Build history of the part. All positions in model axes, mm. A direction names the side the tool comes from. Coordinates: 2 decimals unless noted, no trailing zeros. Order: outer loops, then holes, each group sorted by start corner. A loop starts at its lowest first (then second) coordinate and runs counter-clockwise, first axis right, second up. Notation, with made-up numbers: (64.25, 54.25) - (76.25, 54.25) arc R6 ccw to (76.25, 64.25) - close; hole circle Ø8 at (-5.75, 49.5). An arc over 180 degrees is marked (long way). Write each question's results on one line, items separated by ' | '. Start each with the question number.
from build123d import *

# Parameters (mm, degrees)
SKETCH1_W           = 200
SKETCH1_H           = 78
BOSS_EXTRUDE1_DEPTH = 4
SKETCH2_W           = 35
SKETCH2_H           = 4
CUT_EXTRUDE1_DEPTH  = 4
CUT_EXTRUDE2_DEPTH  = 4


with BuildPart() as part:
    # Sketch1 → Boss-Extrude1 (new body)
    with BuildSketch(Plane.XY):
        with Locations((-100, 39)):
            Rectangle(SKETCH1_W, SKETCH1_H)
    extrude(amount=BOSS_EXTRUDE1_DEPTH)

    # Sketch2 → Cut-Extrude1 (cut)
    with BuildSketch(Plane.XY.offset(4)):
        with Locations((-182.5, 76)):
            Rectangle(SKETCH2_W, SKETCH2_H)
        with Locations((-127.5, 76)):
            Rectangle(SKETCH2_W, SKETCH2_H)
        with Locations((-72.5, 76)):
            Rectangle(SKETCH2_W, SKETCH2_H)
        with Locations((-17.5, 76)):
            Rectangle(SKETCH2_W, SKETCH2_H)
        with Locations((-182.5, 2)):
            Rectangle(SKETCH2_W, SKETCH2_H)
        with Locations((-127.5, 2)):
            Rectangle(SKETCH2_W, SKETCH2_H)
        with Locations((-72.5, 2)):
            Rectangle(SKETCH2_W, SKETCH2_H)
        with Locations((-17.5, 2)):
            Rectangle(SKETCH2_W, SKETCH2_H)
    extrude(amount=-CUT_EXTRUDE1_DEPTH, mode=Mode.SUBTRACT)

    # Sketch4 → Cut-Extrude2 (cut)
    with BuildSketch(Plane.XY.offset(4)):
        Polygon((-125.75, 74), (-129.25, 74), (-129.25, 70.25), (-130.5, 70.25), (-130.5, 67.75), (-129.25, 67.75), (-129.25, 64), (-125.75, 64), (-125.75, 67.75), (-124.5, 67.75), (-124.5, 70.25), (-125.75, 70.25), align=None)
        Polygon((-70.75, 67.75), (-69.5, 67.75), (-69.5, 70.25), (-70.75, 70.25), (-70.75, 74), (-74.25, 74), (-74.25, 70.25), (-75.5, 70.25), (-75.5, 67.75), (-74.25, 67.75), (-74.25, 64), (-70.75, 64), align=None)
    extrude(amount=-CUT_EXTRUDE2_DEPTH, mode=Mode.SUBTRACT)


solid = part.part
Item 1: Which spindle directions (+Z, -Z, +X, -X, +Y, -Y) get a long thin tool onto all of the face, cutting with end or side? Do faces 4 (the flat face through (-165, 76, 2)), 5 (the flat face through (-73, 4, 2)), 6 (the flat face through (-145, 76, 2)). Say none if no direction does.
Item 2: Pull direction X, two halves, no side cores. Call faces 1 (the flat face through (-183, 74, 2)), 2 (the flat face through (-70.75, 66, 2)), 3 (the flat face through (-35, 2, 2)): released by +X, released by -X, zero draft, split by the parting line, or undercut.
Item 3: Slice it at A-A (x = -83). Write the cut outline in (y, z).
Item 4: Probe probe 1 along X at (y, z) = (69, 2.2); probe 2 along Y at (x, z) = (-70.5, 1.1); probe 3 along Y at (x, z) = (-118.5, 0.2). List the from-to ranges inside material, lowest first.
Item 5: Flat gauge pins, fed straight in: P1, Ø1.2, axis at x = -74, z = 3, coming from the -Y side; P2, Ø1.4, axis at x = -70, z = 1.5, coming from the +Y side. Where does each tip first touch, or does it go through?
Resolved:
1) face 4: +Z, -Z, -X, +Y | face 5: +Z, -Z, -Y | face 6: +Z, -Z, +Y
2) face 1: zero draft | face 2: undercut | face 3: released by +X
3) outline: (4, 0) - (74, 0) - (74, 4) - (4, 4) - close
4) probe 1: -200 to -130.5, -124.5 to -75.5, -69.5 to 0 | probe 2: 4 to 67.75, 70.25 to 74 | probe 3: 4 to 74
5) P1: y = 4 | P2: y = 74
